Check sheet for the drawn part. Datum: minimum x, y, z corner. Units: mm. Coordinates: 2 decimals unless noted, no trailing zeros. Loops run counter-clockwise (first coordinate to the right, second up) from the corner with the lowest first, then second, coordinate; pieces in that order, holes last. Notation, with made-up numbers: (-3, 31.5) -> (9, 31.5) arc R20 cw to (9, 56.5) -> close; hole circle Ø9 at (-25, 86). An arc over 180 degrees is marked (long way). Use CSV: the item, a comma, the result in double quotes. Start each with the question number.
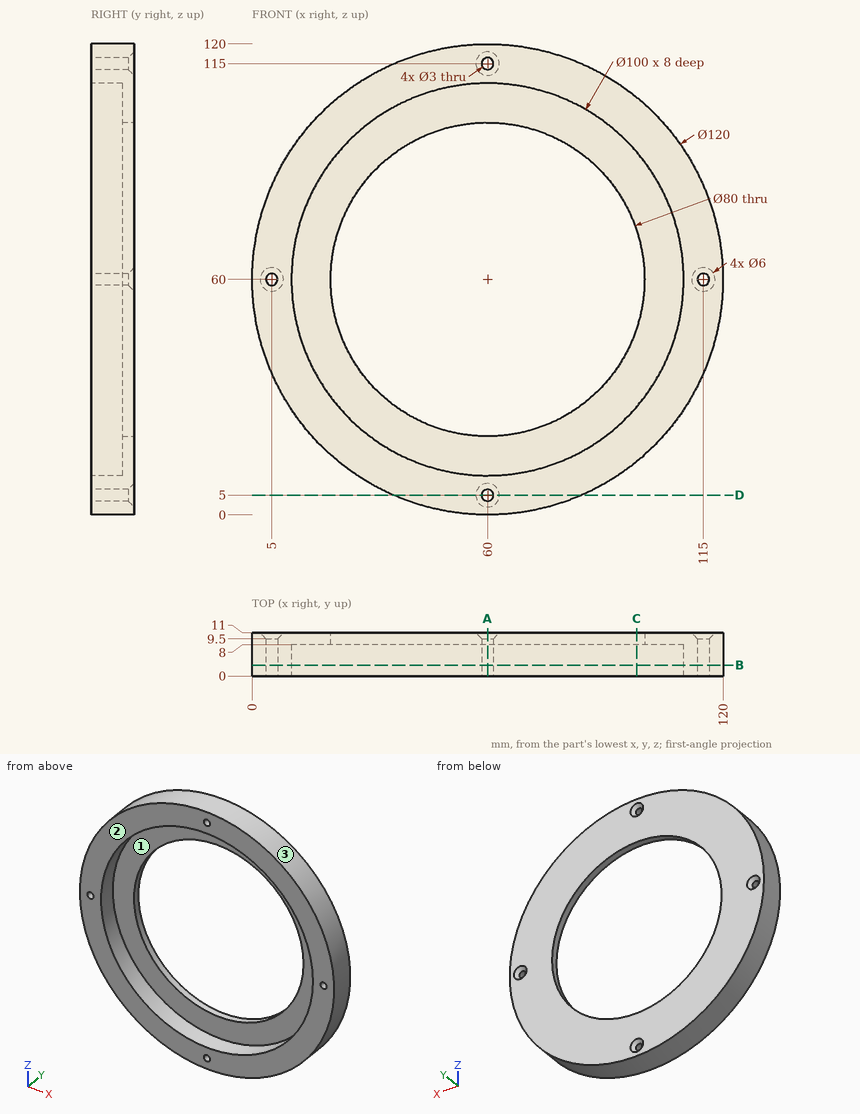
1. Cross-section at D-D, the plane z = 5. Record the boundary of the cut face in (x, y), plus the area to 3 significant figures.
2. Cross-section at B-B, the plane y = 2.75. Record the boundary of the cut face in (x, z).
3. Cross-section at A-A, the plane x = 60. Record the boundary of the cut face in (y, z).
4. Cross-section at C-C, the plane x = 98. Record the boundary of the cut face in (y, z).
5. Scan lines: line 1 (Z direction, x = 60, y = 9.15); line 2 (Z direction, x = 60, y = 4.5); line 3 (X direction, y = 6.75, z = 59). Record each from-to range of solid material in increasing order.
6. Depth check by flat-ended pin: pin 1 (1.5 mm diameter, centred on x = 100.5, z = 65.5, fed in from -Y); pin 2 (2 mm diameter, centred on y = 9, z = 93.5, fed in from +X); pin 3 (5 mm diameter, centred on x = 33.5, y = 7, fed in from -Z). Enter the tip coordinate at first touch or a pass-through.
7. Release check for a two-part mould opening along Z. For the marked faces 1, 2 and 3 record: released by +Z, released by -Z, zero draft, split by the parting line, or undercut.
Solution:
1,outline,"(36.02, 0) -> (58.5, 0) -> (58.5, 9.5) -> (57, 11) -> (36.02, 11) -> close; (61.5, 0) -> (83.98, 0) -> (83.98, 11) -> (63, 11) -> (61.5, 9.5) -> close"
1,area,"492 mm2"
2,outline,"circle Ø120 at (60, 60); hole circle Ø3 at (5, 60); hole circle Ø100 at (60, 60); hole circle Ø3 at (60, 5); hole circle Ø3 at (60, 115); hole circle Ø3 at (115, 60)"
3,outline,"(0, 0) -> (11, 0) -> (11, 2) -> (9.5, 3.5) -> (0, 3.5) -> close; (0, 6.5) -> (9.5, 6.5) -> (11, 8) -> (11, 20) -> (8, 20) -> (8, 10) -> (0, 10) -> close; (0, 110) -> (8, 110) -> (8, 100) -> (11, 100) -> (11, 112) -> (9.5, 113.5) -> (0, 113.5) -> close; (0, 116.5) -> (9.5, 116.5) -> (11, 118) -> (11, 120) -> (0, 120) -> close"
4,outline,"(0, 13.57) -> (11, 13.57) -> (11, 47.51) -> (8, 47.51) -> (8, 27.5) -> (0, 27.5) -> close; (0, 92.5) -> (8, 92.5) -> (8, 72.49) -> (11, 72.49) -> (11, 106.43) -> (0, 106.43) -> close"
5,line 1,"z = 0 to 3.5, 6.5 to 20, 100 to 113.5, 116.5 to 120"
5,line 2,"z = 0 to 3.5, 6.5 to 10, 110 to 113.5, 116.5 to 120"
5,line 3,"x = 0.01 to 3.88, 6.12 to 10.01, 109.99 to 113.88, 116.12 to 119.99"
6,pin 1,"stops at y = 8"
6,pin 2,"stops at x = 110.44"
6,pin 3,"stops at z = 5.01"
7,face 1,"undercut"
7,face 2,"zero draft"
7,face 3,"split by the parting line"
